from build123d import *

# Parameters (mm, degrees)
BOSS_EXTRUDE1_DEPTH          = 5
BOSS_EXTRUDE2_START          = 12
BOSS_EXTRUDE2_DEPTH          = 12
BOSS_EXTRUDE3_START          = 12
BOSS_EXTRUDE3_DEPTH          = 12
SKETCH4_W                    = 4.25
SKETCH4_H                    = 12
CUT_EXTRUDE1_DEPTH           = 44.425942707
SKETCH5_W                    = 4.25
SKETCH5_H                    = 12
CUT_EXTRUDE2_DEPTH           = 44.425942707
BOSS_EXTRUDE4_REACH          = 75.667
F_3_0_3_DIAMETER_HOLE1_D     = 3
F_3_0_3_DIAMETER_HOLE1_DEPTH = 12
SKETCH9_W                    = 1.5
SKETCH9_H                    = 5
F_3_0_3_DIAMETER_HOLE3_D     = 3
F_3_0_3_DIAMETER_HOLE3_DEPTH = 5
F_4_0_4_DIAMETER_HOLE1_D     = 4
F_4_0_4_DIAMETER_HOLE1_DEPTH = 17
FILLET1_R                    = 5
SKETCH15_W                   = 102.81130979
SKETCH15_H                   = 78.647232544
CUT_EXTRUDE3_DEPTH           = 10


with BuildPart() as part:
    # Sketch1 → Boss-Extrude1 (new body)
    with BuildSketch(Plane.XY.offset(8)):
        with BuildLine():
            Line((-6, 57.5), (-6, 56))
            Line((-6, 56), (-27.25, 56))
            ThreePointArc((-27.25, 56), (-33.25, 50), (-27.25, 44))
            Line((-27.25, 44), (-6, 44))
            Line((-6, 44), (-6, 42.5))
            ThreePointArc((-6, 42.5), (0, 36.5), (6, 42.5))
            Line((6, 42.5), (6, 44))
            Line((6, 44), (27.25, 44))
            ThreePointArc((27.25, 44), (33.25, 50), (27.25, 56))
            Line((27.25, 56), (6, 56))
            Line((6, 56), (6, 57.5))
            ThreePointArc((6, 57.5), (0, 63.5), (-6, 57.5))
        make_face()
    extrude(amount=-BOSS_EXTRUDE1_DEPTH)

    # Sketch2 → Boss-Extrude2 (add)
    with BuildSketch(Plane.XY.offset(8).offset(BOSS_EXTRUDE2_START)):
        with BuildLine():
            Line((27.25, 44), (18, 44))
            Line((18, 44), (18, 56))
            Line((18, 56), (27.25, 56))
            ThreePointArc((27.25, 56), (33.25, 50), (27.25, 44))
        make_face()
    extrude(amount=-BOSS_EXTRUDE2_DEPTH)

    # Sketch3 → Boss-Extrude3 (add)
    with BuildSketch(Plane.XY.offset(8).offset(BOSS_EXTRUDE3_START)):
        with BuildLine():
            Line((-27.25, 56), (-18, 56))
            Line((-18, 56), (-18, 44))
            Line((-18, 44), (-27.25, 44))
            ThreePointArc((-27.25, 44), (-33.25, 50), (-27.25, 56))
        make_face()
    extrude(amount=-BOSS_EXTRUDE3_DEPTH)

    # Sketch4 → Cut-Extrude1 (cut, through all)
    with BuildSketch(Plane(origin=(0, 56, 0), x_dir=(-1, 0, 0), z_dir=(0, 1, 0))):
        with Locations((-25.125, 14)):
            Rectangle(SKETCH4_W, SKETCH4_H)
    extrude(amount=-CUT_EXTRUDE1_DEPTH, mode=Mode.SUBTRACT)

    # Sketch5 → Cut-Extrude2 (cut, through all)
    with BuildSketch(Plane(origin=(0, 56, 0), x_dir=(-1, 0, 0), z_dir=(0, 1, 0))):
        with Locations((25.125, 14)):
            Rectangle(SKETCH5_W, SKETCH5_H)
    extrude(amount=-CUT_EXTRUDE2_DEPTH, mode=Mode.SUBTRACT)

    # Sketch6 → Boss-Extrude4 (add, up to next)
    with BuildSketch(Plane.XY.offset(20), mode=Mode.PRIVATE) as boss_extrude4_sk1:
        with BuildLine():
            Line((6, 44), (6, 56))
            Line((6, 56), (3.708099244, 56))
            ThreePointArc((3.708099244, 56), (0, 53.5), (-3.708099244, 56))
            Line((-3.708099244, 56), (-6, 56))
            Line((-6, 56), (-6, 44))
            Line((-6, 44), (-3.708099244, 44))
            ThreePointArc((-3.708099244, 44), (-0.109747314, 46.498494157), (3.620236982, 44.201142026))
            Line((3.620236982, 44.201142026), (6, 44))
        make_face()
    boss_extrude4_tool1 = extrude(boss_extrude4_sk1.sketch, amount=-BOSS_EXTRUDE4_REACH, mode=Mode.PRIVATE) - part.part
    add(boss_extrude4_tool1.solids().sort_by_distance((-0.008751, 50.011684, 20))[0])

    # Ø3.0 (3) Diameter Hole1
    with Locations(Plane.ZY.offset(6)):
        with Locations((18, 50)):
            Hole(F_3_0_3_DIAMETER_HOLE1_D / 2, depth=F_3_0_3_DIAMETER_HOLE1_DEPTH)

    # Sketch9 → Ø3.0 (3) Diameter Hole2 (revolve, cut)
    with BuildSketch(Plane(origin=(23, 50, 18), x_dir=(0, 0, -1), z_dir=(0, 1, 0))):
        with Locations((0.75, 2.5)):
            Rectangle(SKETCH9_W, SKETCH9_H)
    revolve(axis=Axis((29.35, 50, 18), (-1, 0, 0)), mode=Mode.SUBTRACT)

    # Ø3.0 (3) Diameter Hole3
    with Locations(Plane(origin=(-18, 0, 0), x_dir=(0, 0, -1), z_dir=(1, 0, 0))):
        with Locations((-18, 50)):
            Hole(F_3_0_3_DIAMETER_HOLE3_D / 2, depth=F_3_0_3_DIAMETER_HOLE3_DEPTH)

    # Ø4.0 (4) Diameter Hole1
    with Locations(Plane(origin=(0, 0, 3), x_dir=(-1, 0, 0), z_dir=(0, 0, -1))):
        with Locations((0, 57.5), (-27.25, 50), (27.25, 50), (0, 42.5)):
            Hole(F_4_0_4_DIAMETER_HOLE1_D / 2, depth=F_4_0_4_DIAMETER_HOLE1_DEPTH)

    # Fillet1
    # the kernel refuses this fillet: 5 mm, written as the material it takes off along each edge
    with BuildSketch(Plane(origin=(-35.5, 56, 20), x_dir=(0, 0, -1), z_dir=(1, 0, 0))) as fillet1_piece_1_section:
        with BuildLine():
            CenterArc((FILLET1_R, -FILLET1_R), FILLET1_R, 90, 90)
            Line((0, -FILLET1_R), (0, 0))
            Line((0, 0), (FILLET1_R, 0))
        make_face()
    fillet1_piece_1 = extrude(amount=30, mode=Mode.PRIVATE)
    fillet1_piece_1 = split(fillet1_piece_1, bisect_by=Plane(origin=(-27.25, 53.041631107, 19.755841734), z_dir=(1, 0, 0)), keep=Keep.TOP, mode=Mode.PRIVATE)
    add(fillet1_piece_1, mode=Mode.SUBTRACT)
    with BuildSketch(Plane(origin=(35.5, 44, 20), x_dir=(0, 0, -1), z_dir=(-1, 0, 0))) as fillet1_piece_2_section:
        with BuildLine():
            CenterArc((FILLET1_R, -FILLET1_R), FILLET1_R, 90, 90)
            Line((0, -FILLET1_R), (0, 0))
            Line((0, 0), (FILLET1_R, 0))
        make_face()
    fillet1_piece_2 = extrude(amount=30, mode=Mode.PRIVATE)
    fillet1_piece_2 = split(fillet1_piece_2, bisect_by=Plane(origin=(27.25, 46.958368888, 19.755841732), z_dir=(-1, 0, 0)), keep=Keep.TOP, mode=Mode.PRIVATE)
    add(fillet1_piece_2, mode=Mode.SUBTRACT)
    with BuildSketch(Plane(origin=(5.5, 56, 20), x_dir=(0, 0, -1), z_dir=(1, 0, 0))) as fillet1_piece_3_section:
        with BuildLine():
            CenterArc((FILLET1_R, -FILLET1_R), FILLET1_R, 90, 90)
            Line((0, -FILLET1_R), (0, 0))
            Line((0, 0), (FILLET1_R, 0))
        make_face()
    fillet1_piece_3 = extrude(amount=30, mode=Mode.PRIVATE)
    fillet1_piece_3 = split(fillet1_piece_3, bisect_by=Plane(origin=(27.25, 54.883160305, 18.883160305), z_dir=(-1, 0, 0)), keep=Keep.TOP, mode=Mode.PRIVATE)
    add(fillet1_piece_3, mode=Mode.SUBTRACT)
    with BuildSketch(Plane(origin=(-18.5, 44, 20), x_dir=(0, 1, 0), z_dir=(1, 0, 0))) as fillet1_piece_4:
        with BuildLine():
            CenterArc((FILLET1_R, -FILLET1_R), FILLET1_R, 90, 90)
            Line((0, -FILLET1_R), (0, 0))
            Line((0, 0), (FILLET1_R, 0))
        make_face()
    extrude(amount=27.291900756, mode=Mode.SUBTRACT)
    with BuildSketch(Plane(origin=(18.5, 56, 20), x_dir=(0, 0, -1), z_dir=(-1, 0, 0))) as fillet1_piece_5:
        with BuildLine():
            CenterArc((FILLET1_R, FILLET1_R), FILLET1_R, 180, 90)
            Line((0, FILLET1_R), (0, 0))
            Line((0, 0), (FILLET1_R, 0))
        make_face()
    extrude(amount=27.291900756, mode=Mode.SUBTRACT)
    with BuildSketch(Plane(origin=(-5.5, 44, 20), x_dir=(0, 1, 0), z_dir=(-1, 0, 0))) as fillet1_piece_6_section:
        with BuildLine():
            CenterArc((FILLET1_R, FILLET1_R), FILLET1_R, 180, 90)
            Line((0, FILLET1_R), (0, 0))
            Line((0, 0), (FILLET1_R, 0))
        make_face()
    fillet1_piece_6 = extrude(amount=30, mode=Mode.PRIVATE)
    fillet1_piece_6 = split(fillet1_piece_6, bisect_by=Plane(origin=(-27.25, 45.116839695, 18.883160305), z_dir=(1, 0, 0)), keep=Keep.TOP, mode=Mode.PRIVATE)
    add(fillet1_piece_6, mode=Mode.SUBTRACT)

    # Sketch15 → Cut-Extrude3 (cut)
    with BuildSketch(Plane(origin=(0, 0, 3), x_dir=(-1, 0, 0), z_dir=(0, 0, -1))):
        with Locations((1.036291242, 56.487506321)):
            Rectangle(SKETCH15_W, SKETCH15_H)
    extrude(amount=CUT_EXTRUDE3_DEPTH, mode=Mode.SUBTRACT)


solid = part.part
Source: CAD feature listing. Evaluate the final solid. Frame: model axes, mm. A direction names the side the tool comes from. Coordinates: 2 decimals unless noted, no trailing zeros. Loops run counter-clockwise (first coordinate to the right, second up) from the corner with the lowest first, then second, coordinate; pieces in that order, holes last. Notation, with made-up numbers: (41, 17.5) -> (94, 17.5) arc R21 ccw to (94, 27.5) -> close; hole circle Ø2 at (17.25, 28.25). An arc over 180 degrees is marked (long way). Answer in a Markdown table with one row per item. Add a question column.
Q1. Section B-B on z = 14.25. Return the cut outline in (x, y).
Q2. Contact query for flat-ended pins moving along their axis: pin 1 Ø1.3 at (x, y) = (24.5, 50.5) entering from +Z; pin 2 Ø4.5 at (y, z) = (45, 16.5) entering from +X; pin 3 Ø9.5 at (x, z) = (-20, 7) entering from +Y. Output: stop coordinate, or through.
Q3. Pull-direction query (X, two-part tool) for faces 1 (the face through (18, 50, 13)), 2 (the face through (30, 50, 20)), 3 (the face through (33.25, 50.13, 11.62)); classes: pulls with the +X half, pulls with the -X half, needs draft (parallel to the pull), parting line crosses it, or undercut.
Q4. Section C-C on z = 5. Return the cut outline in (x, y), and give its area (3 significant figures).
Q5. Ray query, line 1 along Y through (x, z) = (0, 4.45); line 2 along Z through (x, y) = (20.4, 50); line 3 along Y through (x, z) = (2.5, 18). Return the intervals inside material, ascending.
Q6. Section A-A on x = 0. Return the cut outline in (y, z), and give its area (3 significant figures).
Q7. Reachability of faces 4 (the face through (0, 60, 8)), 5 (the face through (16, 56, 6)), 6 (the face through (-27.25, 54, 14)) from +Z, -Z, +X, -X, +Y, -Y: full face, straight path, thin tool, end or side. Return the list, or none.
Q8. Section D-D on x = 14.5. Return the cut outline in (y, z).
Computed values:
| question | item | result |
|---|---|---|
| 1 | outline | (-27.25, 44) -> (-27.25, 48) arc R2 cw to (-27.25, 52) -> (-27.25, 56) arc R6 ccw to start; (-23, 44) -> (-18, 44) -> (-18, 56) -> (-23, 56) -> close; (-6, 44) -> (-3.71, 44) arc R4 cw to (3.62, 44.2) -> (6, 44) -> (6, 56) -> (3.71, 56) arc R4 cw to (-3.71, 56) -> (-6, 56) -> close; (18, 44) -> (23, 44) -> (23, 56) -> (18, 56) -> close; (27.25, 44) arc R6 ccw to (27.25, 56) -> (27.25, 52) arc R2 cw to (27.25, 48) -> close |
| 2 | pin 1 | stops at z = 8 |
| 2 | pin 2 | stops at x = 32.58 |
| 2 | pin 3 | stops at y = 56 |
| 3 | face 1 | undercut |
| 3 | face 2 | needs draft |
| 3 | face 3 | pulls with the +X half |
| 4 | outline | (-27.25, 44) -> (-6, 44) -> (-6, 42.5) arc R6 ccw to (6, 42.5) -> (6, 44) -> (27.25, 44) arc R6 ccw to (27.25, 56) -> (6, 56) -> (6, 57.5) arc R6 ccw to (-6, 57.5) -> (-6, 56) -> (-27.25, 56) arc R6 ccw to start; hole circle Ø4 at (-27.25, 50); hole circle Ø4 at (0, 42.5); hole circle Ø4 at (0, 57.5); hole circle Ø4 at (27.25, 50) |
| 4 | area | 866 mm^2 |
| 5 | line 1 | y = 36.5 to 40.5, 44.5 to 55.5, 59.5 to 63.5 |
| 5 | line 2 | z = 3 to 16.5, 19.5 to 20 |
| 5 | line 3 | y = 45.62 to 48.5, 51.5 to 54.38 |
| 6 | outline | (36.5, 3) -> (40.5, 3) -> (40.5, 8) -> (36.5, 8) -> close; (44.5, 3) -> (55.5, 3) -> (55.5, 8) -> (53.5, 8) -> (53.5, 19.33) arc R5 ccw to (51, 20) -> (49, 20) arc R5 ccw to (46.5, 19.33) -> (46.5, 8) -> (44.5, 8) -> close; (59.5, 3) -> (63.5, 3) -> (63.5, 8) -> (59.5, 8) -> close; hole circle Ø3 at (50, 18) |
| 6 | area | 171 mm^2 |
| 7 | face 4 | +Z, +Y |
| 7 | face 5 | +Z, -Z, +X, +Y |
| 7 | face 6 | +Z, +Y, -Y |
| 8 | outline | (44, 3) -> (56, 3) -> (56, 8) -> (44, 8) -> close |
